Here's the drawing with two shaded views (mm, measured from the low corner). I have some questions. Coordinates: 2 decimals unless noted, no trailing zeros. Loops run counter-clockwise (first coordinate to the right, second up) from the corner with the lowest first, then second, coordinate; pieces in that order, holes last.
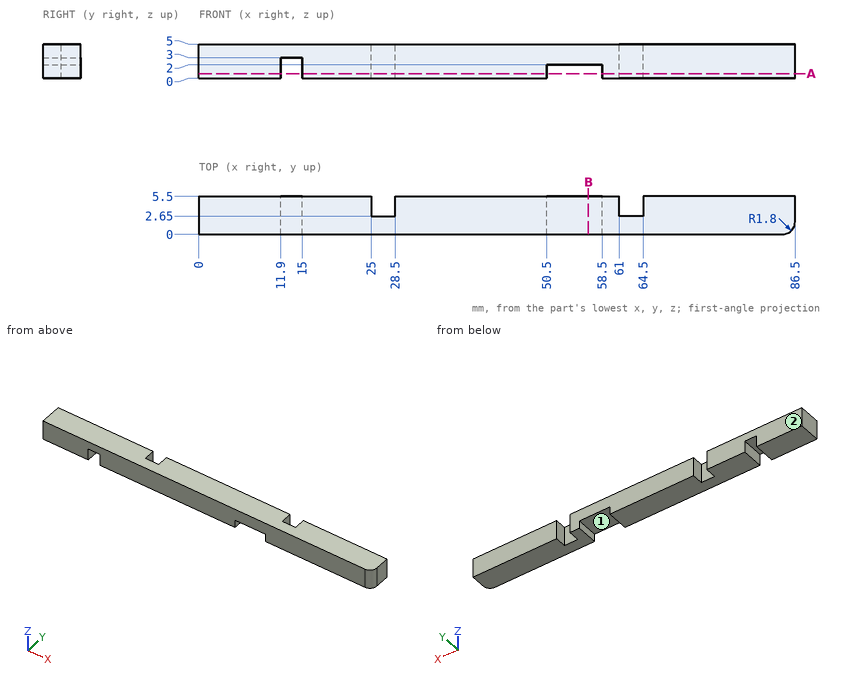
(1) I'm going to push flat-ended pins straight in: pin 1 (1.6 mm diameter, centred on x = 54, y = 2.5, fed in from -Z); pin 2 (2 mm diameter, centred on y = 2.5, z = 1, fed in from -X); pin 3 (1 mm diameter, centred on x = 26, z = 2, fed in from +Y). Where does each tip first touch, or does it pass through?
Check values:
pin 1: stops at z = 2
pin 2: stops at x = 0
pin 3: stops at y = 2.65
(2) If I drill on probe 1 along X at (y, z) = (5, 0.9); probe 2 along X at (y, z) = (4.05, 4.4); probe 3 along X at (y, z) = (3.1, 2.1), over which ranges is the centre line in solid material (lowest first)?
Check values:
probe 1: x = 0 to 11.9, 15 to 25, 28.5 to 50.5, 58.5 to 61, 64.5 to 86.5
probe 2: x = 0 to 25, 28.5 to 61, 64.5 to 86.5
probe 3: x = 0 to 11.9, 15 to 25, 28.5 to 61, 64.5 to 86.5
(3) If we mould it in two halves opening along X, with no side actions, what happens to the marked faces 1 and 2? For each: released by +X, released by -X, zero draft, split by the parting line, or undercut.
Check values:
face 1: undercut
face 2: zero draft
(4) I want a section at A-A on z = 0.7. Write out the boundary of the cut face in (x, y).
Check values:
outline: (0, 0) - (11.9, 0) - (11.9, 5.5) - (0, 5.5) - close; (15, 0) - (50.5, 0) - (50.5, 5.5) - (28.5, 5.5) - (28.5, 2.65) - (25, 2.65) - (25, 5.5) - (15, 5.5) - close; (58.5, 0) - (84.7, 0) arc R1.8 ccw to (86.5, 1.8) - (86.5, 5.5) - (64.5, 5.5) - (64.5, 2.65) - (61, 2.65) - (61, 5.5) - (58.5, 5.5) - close
(5) I want a section at B-B on x = 56.5. Write out the boundary of the cut face in (y, z).
Check values:
outline: (0, 2) - (5.5, 2) - (5.5, 5) - (0, 5) - close
